Geometry check sheet. Reference: drawing and pictorial views, mm from the part's lowest x, y, z. Round coordinates to 2 decimals unless told otherwise and drop trailing zeros. Order: outer loops, then holes, each group sorted by start corner. A loop starts at its lowest first (then second) coordinate and runs counter-clockwise, first axis right, second up.
Q1. Cross-section at A-A on x = 7. Record the cut outline in (y, z).
Q2. Cross-section at B-B on z = 77. Record the cut outline in (x, y).
Q3. Scan lines: probe 1 along Y at (x, z) = (10, 76); probe 2 along Y at (x, z) = (1.75, 12). Record each from-to range of solid material in increasing order.
Q4. Depth check by flat-ended pin: P1, Ø6, axis at x = 4.5, z = 10.5, coming from the -Y side; P2, Ø1.5, axis at x = 5.5, z = 7, coming from the -Y side; P3, Ø4, axis at x = 4, y = 7.5, coming from the -Z side. Enter the tip coordinate at first touch or a pass-through.
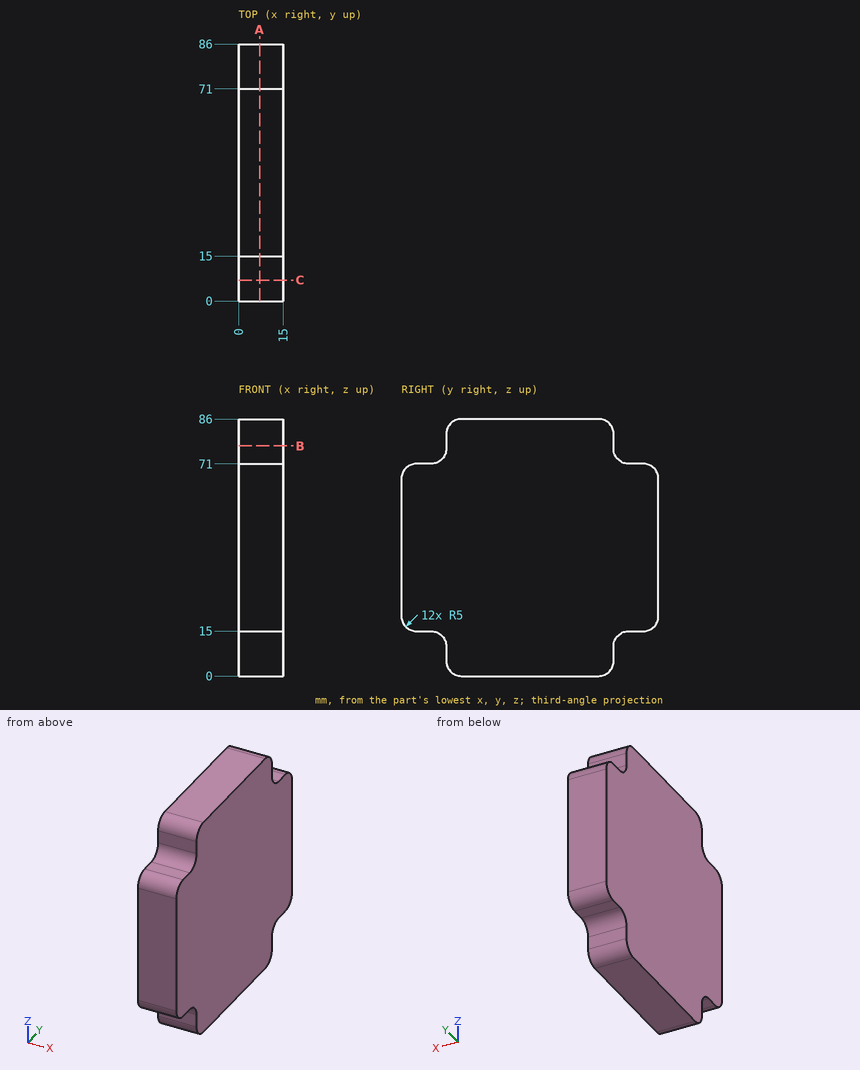
Results found:
1. outline: (0, 20) arc R5 ccw to (5, 15) - (10, 15) arc R5 cw to (15, 10) - (15, 5) arc R5 ccw to (20, 0) - (66, 0) arc R5 ccw to (71, 5) - (71, 10) arc R5 cw to (76, 15) - (81, 15) arc R5 ccw to (86, 20) - (86, 66) arc R5 ccw to (81, 71) - (76, 71) arc R5 cw to (71, 76) - (71, 81) arc R5 ccw to (66, 86) - (20, 86) arc R5 ccw to (15, 81) - (15, 76) arc R5 cw to (10, 71) - (5, 71) arc R5 ccw to (0, 66) - close
2. outline: (0, 15) - (15, 15) - (15, 71) - (0, 71) - close
3. probe 1: y = 15 to 71
3. probe 2: y = 14.58 to 71.42
4. P1: stops at y = 13.57
4. P2: stops at y = 15
4. P3: stops at z = 15
